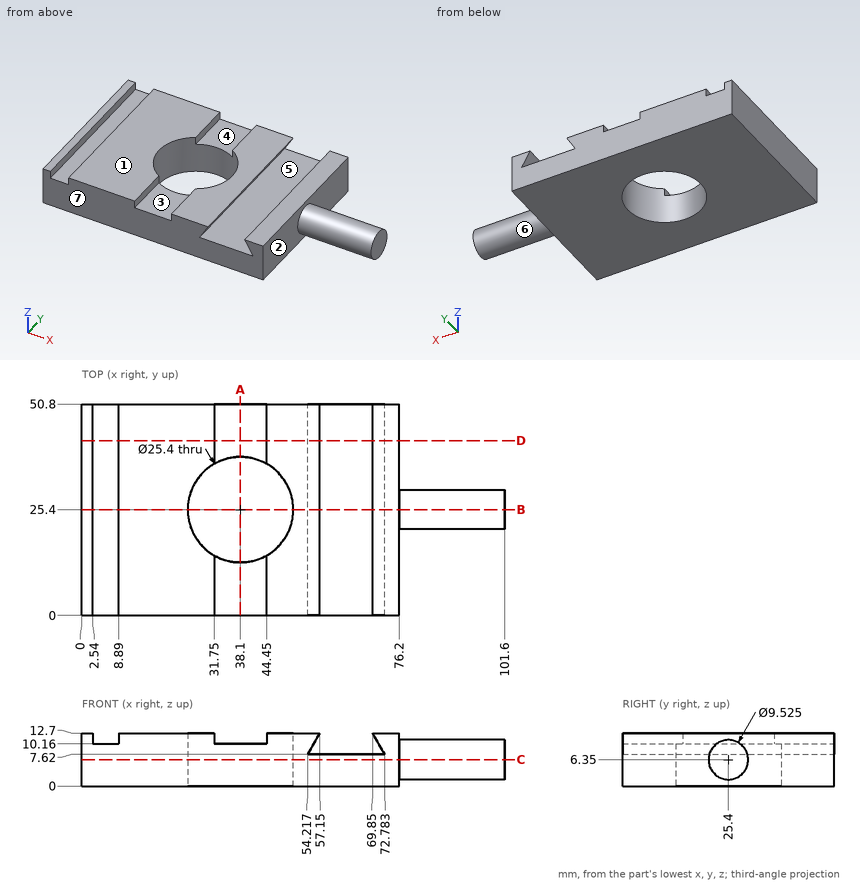
Part print with two shaded views. Sizes in mm from the minimum x, y, z corner. A direction names the side the tool comes from. Give positions to 0.01 mm unless a question says otherwise; leave off trailing zeros. Order: outer loops, then holes, each group sorted by start corner. A loop starts at its lowest first (then second) coordinate and runs counter-clockwise, first axis right, second up. Notation, with made-up numbers: M 42.25,-29 L 90.25,-29 A6 ccw 90.25,-22 Z; hole C 28.5,13.5 d3. An arc over 180 degrees is marked long. Put each result on its own line as item: value.
Item 1: Drop flat-ended pins along their axis: pin 1 Ø3 at (y, z) = (8.5, 12) entering from +X; pin 2 Ø6 at (x, z) = (80, 3.5) entering from +Y; pin 3 Ø10 at (x, y) = (39, 6.5) entering from +Z. Give the stop position or say it passes through.
Results are:
pin 1: x = 76.2
pin 2: y = 30.16
pin 3: z = 10.16
Item 2: Wall check: probe 1 along X at (y, z) = (25.4, 5); probe 2 along Y at (x, z) = (38.1, 4.75); probe 3 along X at (y, z) = (27, 9.25). Give the ranges that are in metal, low to high.
Results are:
probe 1: 0 to 25.4, 50.8 to 101.6
probe 2: 0 to 12.7, 38.1 to 50.8
probe 3: 0 to 25.5, 50.7 to 55.16, 71.84 to 101.6
Item 3: Cut at C-C on z = 6.35. Write the cut outline in (x, y), then the cut area to 3 significant figures.
Results are:
outline: M 0,0 L 76.2,0 L 76.2,20.64 L 101.6,20.64 L 101.6,30.16 L 76.2,30.16 L 76.2,50.8 L 0,50.8 Z; hole C 38.1,25.4 d25.4
area: 3,610 mm2
Item 4: Pull direction X, two halves, no side cores. Call the marked faces 1, 2, 3 and 4: +X half, -X half, draft (parallel to the pull), parting line (faces both ways), or undercut.
Results are:
face 1: draft
face 2: +X half
face 3: undercut
face 4: undercut
Item 5: Cut at A-A on x = 38.1. Write the cut outline in (y, z), then the cut area to 3 significant figures.
Results are:
outline: M 0,0 L 12.7,0 L 12.7,10.16 L 0,10.16 Z; M 38.1,0 L 50.8,0 L 50.8,10.16 L 38.1,10.16 Z
area: 258 mm2
Item 6: Which spindle directions (+Z, -Z, +X, -X, +Y, -Y) get a long thin tool onto all of the face, cutting with end or side? Do the marked faces 5, 6 and 7. Say none if no direction does.
Results are:
face 5: +Y, -Y
face 6: +X
face 7: +Z, -Z, +X, -X, -Y
Item 7: Cut at D-D on y = 42. Write the cut outline in (x, z).
Results are:
outline: M 0,0 L 76.2,0 L 76.2,12.7 L 69.85,12.7 L 72.78,7.62 L 54.22,7.62 L 57.15,12.7 L 44.45,12.7 L 44.45,10.16 L 31.75,10.16 L 31.75,12.7 L 8.89,12.7 L 8.89,10.16 L 2.54,10.16 L 2.54,12.7 L 0,12.7 Z
Item 8: Cut at B-B on y = 25.4. Write the cut outline in (x, z), then the cut area to 3 significant figures.
Results are:
outline: M 0,0 L 25.4,0 L 25.4,12.7 L 8.89,12.7 L 8.89,10.16 L 2.54,10.16 L 2.54,12.7 L 0,12.7 Z; M 50.8,0 L 76.2,0 L 76.2,1.59 L 101.6,1.59 L 101.6,11.11 L 76.2,11.11 L 76.2,12.7 L 69.85,12.7 L 72.78,7.62 L 54.22,7.62 L 57.15,12.7 L 50.8,12.7 Z
area: 792 mm2
